Study the drawing (mm; zero at the part's minimum x, y, z) and answer. A direction names the side the tool comes from. Coordinates: 2 decimals unless noted, no trailing zeros. Order: outer loops, then holes, each group sorted by start corner. A loop starts at its lowest first (then second) coordinate and runs counter-clockwise, first axis right, second up. Notation, with made-up numbers: (73, 17) -> (90, 17) arc R13 cw to (90, 35) -> close; hole circle Ø10 at (-26, 6.25). An arc over 180 degrees is marked (long way). Answer as CSV lines item,"result". Start each with the question number.
Item 1: For a pull along X with two mould halves and no side action, classify the marked faces 1, 2 and 3 as pulls with the +X half, pulls with the -X half, needs draft (parallel to the pull), parting line crosses it, or undercut.
Item 2: Straight lines are drawn through the part: L1, parallel to X at y = 5.75, z = 4.5 (1 decimal); L2, parallel to X at y = 7.75, z = 2 (1 decimal); L3, parallel to Y at x = 35.5, z = 1.5. For each, find the intervals that lie inside material, in ascending order.
Item 3: This flat-tipped pin is pushed along its axis until it touches: pin 1 Ø3 at (x, z) = (46, 6) entering from +Y (1 decimal). Where does it stop, or does it pass through?
Item 4: Section D-D (x = 33) is taken. Write down the section's boundary in (y, z).
Item 5: Section A-A (y = 5.75) is taken. Count the separate pieces of the cut face and the enclosed holes in it, then the cut area to 3 significant figures.
Item 6: Which of the six approach directions +Z, -Z, +X, -X, +Y, -Y give full straight-line access (tool end or side, diameter ignored) to the marked faces 4 and 5?
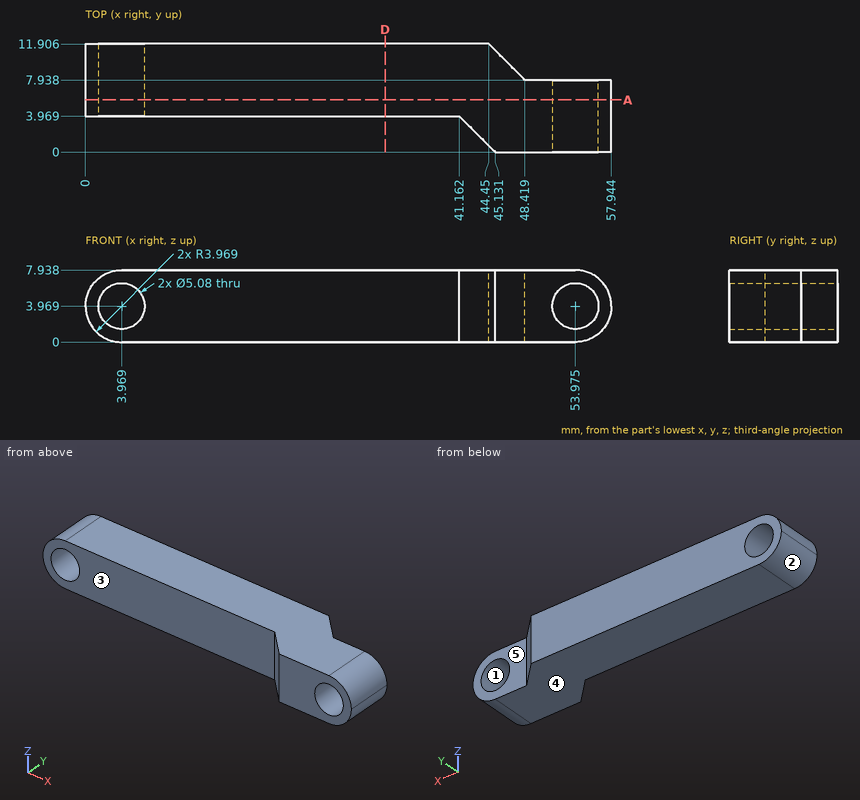
Checked values:
1,face 1,"undercut"
1,face 2,"pulls with the -X half"
1,face 3,"needs draft"
2,L1,"x = 0 to 1.5, 6.5 to 51.5, 56.5 to 57.9"
2,L2,"x = 0.5 to 2.4, 5.6 to 52.4, 55.6 to 57.4"
2,L3,"y = 3.97 to 11.91"
3,pin 1,"stops at y = 11.9"
4,outline,"(3.97, 0) -> (11.91, 0) -> (11.91, 7.94) -> (3.97, 7.94) -> close"
5,separate pieces,"1"
5,enclosed holes,"2"
5,area,"406 mm^2"
6,face 4,"-Z, +X, -X, +Y, -Y"
6,face 5,"+Z, -Z, +X, +Y"
